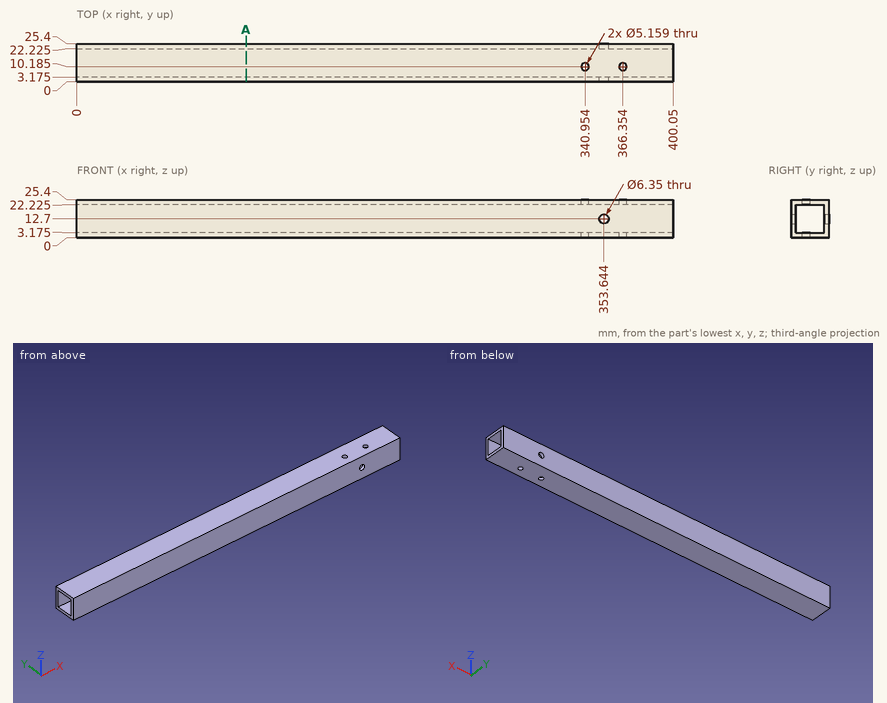
Design review of the part shown in the three views and the two pictorial views. Dimensions are in mm from the part's minimum x, y and z. Give positions to 0.01 mm unless a question says otherwise; leave off trailing zeros. Write each loop counter-clockwise with the first axis right and the second up, starting at its lowest first coordinate (ties: lowest second). Pieces come first, ordered by that corner, then holes. Notation, with made-up numbers: (74.5, -25) - (133.5, -25) arc R30 ccw to (133.5, 13) - close; hole circle Ø11 at (64.25, -27). An arc over 180 degrees is marked (long way). Return JSON: item names as keys, results as strings. Group by question number.
(1) We need section A-A, the plane x = 113.5. Give the boundary of the cut face in (y, z) (1 decimal).
(2) Insertion check: pin 1 (4.5 mm diameter, centred on x = 366.35, y = 10.19, fed in from -Z); pin 2 (6 mm diameter, centred on x = 165, z = 20.5, fed in from -Y). Each pin has a flat end and moves straight along its axis. Give the tip position at first contact, or say it passes through.
(3) To check wall thickness, follow probe 1 along Z at (x, y) = (29.5, 21.5) (1 decimal). State the ranges of the line that lie inside material, in increasing order.
Reported:
{
 "1": {"outline": "(0, 0) - (25.4, 0) - (25.4, 25.4) - (0, 25.4) - close; hole (3.2, 3.2) - (22.2, 3.2) - (22.2, 22.2) - (3.2, 22.2) - close"},
 "2": {"pin 1": "passes through", "pin 2": "stops at y = 0"},
 "3": {"probe 1": "z = 0 to 3.2, 22.2 to 25.4"}
}
